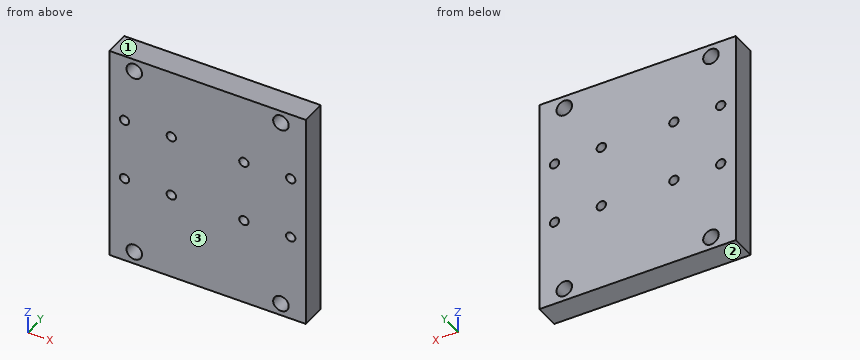
Autodesk Inventor part; units mm, degrees
ref_plane "YZ Plane" through (0, 0, 0) normal (1, 0, 0) x (0, 1, 0)
ref_plane "XZ Plane" through (0, 0, 0) normal (0, 1, 0) x (-1, 0, 0)
ref_plane "XY Plane" through (0, 0, 0) normal (0, 0, 1) x (1, 0, 0)
sketch "Sketch1" plane through (0, 0, 0) normal (0, 1, 0) x (-1, 0, 0)
  line L0 (0, 0) -> (63, 0)
  line L1 (63, 0) -> (63, -70)
  line L2 (63, -70) -> (0, -70)
  line L3 (0, -70) -> (0, 0)
  dimension "d0" = 70
  dimension "d1" = 63
extrude "Extrusion1" add sketch "Sketch1" along normal blind 8
sketch "Sketch2" plane through (0, 8, 0) normal (0, 1, 0) x (1, 0, 0)
  line L0 (0, 70) -> (-63, 70)
  line L1 (-63, 70) -> (-63, 0)
  line L2 (0, 0) -> (0, 70)
  point P0 (-58.125, 42)
  point P1 (-43.125, 42)
  point P2 (-58.125, 22)
  point P3 (-43.125, 22)
  point P4 (-19.875, 42)
  point P5 (-19.875, 22)
  point P6 (-4.875, 42)
  point P7 (-4.875, 22)
  dimension "d4" = 70
  dimension "d5" = 63
  dimension "d8" = 15
  dimension "d11" = 20
  dimension "d18" = 20
  dimension "d21" = 15
  dimension "d24" = 23.25
  dimension "d25" = 0
  dimension "d26" = 28
  dimension "d27" = 53.25
  dimension "d28" = -4.875
hole "Hole1" at (-58.125, 8, -42) at (-43.125, 8, -42) at (-58.125, 8, -22) at (-43.125, 8, -22) at (-19.875, 8, -42) at (-19.875, 8, -22) at (-4.875, 8, -42) at (-4.875, 8, -22) direction (0, -1, 0) diameter 3 end through all
sketch "Sketch3" plane through (0, 8, 0) normal (0, 1, 0) x (1, 0, 0)
  line L0 (0, 0) -> (0, 70)
  line L1 (-63, 0) -> (0, 0)
  point P0 (-8, 4)
  point P1 (-55, 4)
  point P2 (-8, 66)
  point P3 (-55, 66)
  dimension "d38" = 47
  dimension "d41" = 62
  dimension "d44" = 63
  dimension "d45" = 70
  dimension "d46" = 4
  dimension "d47" = 8
hole "Hole2" at (-8, 8, -4) at (-55, 8, -4) at (-8, 8, -66) at (-55, 8, -66) direction (0, -1, 0) diameter 5 end through all
equation "\"d34\" = Thickness"
equation "\"d53\" = Thickness"
equation "\"BendRadius\" = Thickness"
equation "\"BendReliefWidth\" = Thickness"
equation "\"BendReliefDepth\" = 0.5 * Thickness"
equation "\"CornerReliefSize\" = 4 * Thickness"
equation "\"MinimumRemnant\" = 2 * Thickness"
equation "\"TransitionRadius\" = BendRadius"
equation "\"JacobiRadiusSize\" = BendRadius"
equation "\"GapSize\" = Thickness"
properties part number "Lateral da caixa de sustentação" material "Aluminum 6061"
Here's how the part is built. I have some questions about the finished solid (model axes, mm). Face numbers are marked on the shaded views. Round coordinates to 2 decimals unless told otherwise and drop trailing zeros. Write each loop counter-clockwise with the first axis right and the second up, starting at its lowest first coordinate (ties: lowest second). Pieces come first, ordered by that corner, then holes. Notation, with made-up numbers: M 10.25,48 L 38.25,48 A21 cw 38.25,69 Z; hole C 58.5,-39.5 d11. An arc over 180 degrees is marked long. Answer as CSV lines item,"result". Start each with the question number.
1. Suppose I cut it at D-D on y = 1.25. Count the separate pieces of the cut face and the enclosed holes in it, then the cut area to 3 significant figures.
2. Suppose I cut it at A-A on z = -42. Write out the boundary of the cut face in (x, y) (3 decimals).
3. Thinking about a two-plate mould opening in Z: for the marked faces 1, 2 and 3, which applies, released by +Z, released by -Z, zero draft, split by the parting line, or undercut?
4. I need wall thicknesses on probe 1 along X at (y, z) = (1.5, -42) (3 decimals); probe 2 along Z at (x, y) = (-55, 4); probe 3 along Z at (x, y) = (-43, 3.25). Which ranges of each line are inside material? Lowest first, please.
5. Suppose I cut it at C-C on x = -55. Write out the boundary of the cut face in (y, z), then the cut area to 3 significant figures.
6. Suppose I cut it at B-B on z = -66. Write out the boundary of the cut face in (x, y), then the cut area to 3 significant figures.
Check result:
1,separate pieces,"1"
1,enclosed holes,"12"
1,area,"4,270 mm2"
2,outline,"M -63,0 L -59.625,0 L -59.625,8 L -63,8 Z; M -56.625,0 L -44.625,0 L -44.625,8 L -56.625,8 Z; M -41.625,0 L -21.375,0 L -21.375,8 L -41.625,8 Z; M -18.375,0 L -6.375,0 L -6.375,8 L -18.375,8 Z; M -3.375,0 L 0,0 L 0,8 L -3.375,8 Z"
3,face 1,"released by +Z"
3,face 2,"released by -Z"
3,face 3,"zero draft"
4,probe 1,"x = -63 to -59.625, -56.625 to -44.625, -41.625 to -21.375, -18.375 to -6.375, -3.375 to 0"
4,probe 2,"z = -70 to -68.5, -63.5 to -6.5, -1.5 to 0"
4,probe 3,"z = -70 to -43.49, -40.51 to -23.49, -20.51 to 0"
5,outline,"M 0,-70 L 8,-70 L 8,-68.5 L 0,-68.5 Z; M 0,-63.5 L 8,-63.5 L 8,-6.5 L 0,-6.5 Z; M 0,-1.5 L 8,-1.5 L 8,0 L 0,0 Z"
5,area,"480 mm2"
6,outline,"M -63,0 L -57.5,0 L -57.5,8 L -63,8 Z; M -52.5,0 L -10.5,0 L -10.5,8 L -52.5,8 Z; M -5.5,0 L 0,0 L 0,8 L -5.5,8 Z"
6,area,"424 mm2"
